Work out the finished part from the listing and answer in its coordinate system (mm). A direction names the side the tool comes from. Give positions to 0.01 mm unless a question says otherwise; leave off trailing zeros. Order: outer loops, then holes, each group sorted by start corner. A loop starts at its lowest first (then second) coordinate and runs counter-clockwise, first axis right, second up. Notation, with made-up numbers: M 31.25,-20.75 L 60.25,-20.75 A4 ccw 60.25,-15.75 Z; hole C 84,88 d6. An arc over 180 degrees is marked long. One line per item, written item: value.
from build123d import *

# Parameters (mm, degrees)
PAD_DEPTH     = 10
SKETCH001_W   = 27
SKETCH001_H   = 21
SKETCH001_W_2 = 50
SKETCH001_H_2 = 10
POCKET_DEPTH  = 10.001


with BuildPart() as part:
    # Sketch → Pad (new body)
    with BuildSketch(Plane(origin=(0, 0, 0), x_dir=(-1, 0, 0), z_dir=(0, 1, 0))):
        Polygon((0, 0), (560, 0), (570, 0), (570, 50), (560, 50), (560, 323), (570, 323), (570, 373), (560, 373), (560, 646), (570, 646), (570, 696), (560, 696), (0, 696), (-10, 696), (-10, 646), (0, 646), (0, 373), (-10, 373), (-10, 323), (0, 323), (0, 50), (-10, 50), (-10, 0), align=None)
    extrude(amount=PAD_DEPTH)

    # Sketch001 → Pocket (cut, through all)
    with BuildSketch(Plane(origin=(0, 10, 0), x_dir=(-1, 0, 0), z_dir=(0, 1, 0))):
        with BuildLine():
            Line((108.335, 536.67), (451.675, 536.67))
            ThreePointArc((466.675, 521.67), (462.281602, 532.276602), (451.675, 536.67))
            Line((466.675, 521.67), (466.675, 229.67))
            ThreePointArc((451.675, 214.67), (462.281602, 219.063398), (466.675, 229.67))
            Line((451.675, 214.67), (108.335, 214.67))
            ThreePointArc((93.335, 229.67), (97.728398, 219.063398), (108.335, 214.67))
            Line((93.335, 229.67), (93.335, 521.67))
            ThreePointArc((108.335, 536.67), (97.728398, 532.276602), (93.335, 521.67))
        make_face()
        with BuildLine():
            Line((60, 30), (75, 30))
            Line((80.3, 35.5), (75, 30))
            Line((80.3, 47), (80.3, 35.5))
            ThreePointArc((80.3, 47), (79.86066, 48.06066), (78.8, 48.5))
            Line((78.8, 48.5), (56.2, 48.5))
            ThreePointArc((56.2, 48.5), (55.13934, 48.06066), (54.7, 47))
            Line((54.7, 47), (54.7, 35.5))
            Line((54.7, 35.5), (60, 30))
        make_face()
        with Locations((67.5, 67)):
            Rectangle(SKETCH001_W, SKETCH001_H)
        with Locations((125, 5)):
            Rectangle(SKETCH001_W_2, SKETCH001_H_2)
        with Locations((435, 5)):
            Rectangle(SKETCH001_W_2, SKETCH001_H_2)
    extrude(amount=-POCKET_DEPTH, mode=Mode.SUBTRACT)


solid = part.part
(1) Which of the six approach directions +Z, -Z, +X, -X, +Y, -Y give full straight-line access (tool end or side, diameter ignored) to faces 3 (the cylindrical face through (-462.398, 5.07, 532.159)), 4 (the flat face through (-276, 10, 198))?
Findings:
face 3: +Y, -Y
face 4: +Z, -Z, +X, -X, +Y
(2) Section C-C, the plane z = 99 is taken. Give the vertices of the cut face in (x, y), then the cut area to 3 significant figures.
Findings:
outline: M -560,0 L 0,0 L 0,10 L -560,10 Z
area: 5,600 mm^2
(3) Section B-B, the plane y = 6.5 is taken. Give the number of separate pieces and of enclosed holes in the cut face, then the cut area to 3 significant figures.
Findings:
separate pieces: 1
enclosed holes: 3
area: 271,000 mm^2
(4) Determine the mould class of faces 1 (the cylindrical face through (-462.164, 5.07, 218.947)), 2 (the flat face through (-276, 0, 198)) for opening direction X: pulls with the +X half, pulls with the -X half, needs draft (parallel to the pull), parting line crosses it, or undercut.
Findings:
face 1: undercut
face 2: needs draft
(5) Find the intervals of material crossed by probe 1 along Z at (x, y) = (-301, 3.25); probe 2 along X at (y, z) = (4.25, 260.5) (3 decimals); probe 3 along X at (y, z) = (8.25, 355) (3 decimals), in increasing order. Write a range as from..to.
Findings:
probe 1: z = 0..214.67, 536.67..696
probe 2: x = -560..-466.675, -93.335..0
probe 3: x = -570..-466.675, -93.335..10
(6) Section A-A, the plane x = -363 is taken. Give the vertices of the cut face in (y, z).
Findings:
outline: M 0,0 L 10,0 L 10,214.67 L 0,214.67 Z; M 0,536.67 L 10,536.67 L 10,696 L 0,696 Z
(7) Given P1, Ø5, axis at y = 6.5, z = 320, coming from the -X side, flat-ended and moving along its own axis, determine where the tip first touches the part or whether it passes through.
Findings:
P1: stops at x = -560
